Work out the finished part from the listing and answer in its coordinate system (mm). Coordinates: 2 decimals unless noted, no trailing zeros. Loops run counter-clockwise (first coordinate to the right, second up) from the corner with the lowest first, then second, coordinate; pieces in that order, holes last.
```python
from build123d import *

# Parameters (mm, degrees)
F1_DEPTH = 4.7625


with BuildPart() as f1:
    # F0 (on Front) → F1 (new body)
    with BuildSketch(Plane.XZ):
        with BuildLine():
            Line((-57.785, 0), (-2.54, 0))
            ThreePointArc((-2.54, 0), (-0.743949, 0.743949), (0, 2.54))
            Line((0, 2.54), (0, 35.56))
            ThreePointArc((0, 35.56), (-0.743949, 37.356051), (-2.54, 38.1))
            Line((-2.54, 38.1), (-10.16, 38.1))
            ThreePointArc((-10.16, 38.1), (-11.956051, 37.356051), (-12.7, 35.56))
            Line((-12.7, 35.56), (-12.7, 12.7))
            Line((-12.7, 12.7), (-17.4625, 12.7))
            Line((-17.4625, 12.7), (-17.4625, 35.56))
            ThreePointArc((-17.4625, 35.56), (-18.206449, 37.356051), (-20.0025, 38.1))
            Line((-20.0025, 38.1), (-40.3225, 38.1))
            ThreePointArc((-40.3225, 38.1), (-42.118551, 37.356051), (-42.8625, 35.56))
            Line((-42.8625, 35.56), (-42.8625, 12.7))
            Line((-42.8625, 12.7), (-47.625, 12.7))
            Line((-47.625, 12.7), (-47.625, 63.5))
            Line((-47.625, 63.5), (-47.625, 69.85))
            ThreePointArc((-47.625, 69.85), (-49.484872, 74.340128), (-53.975, 76.2))
            Line((-53.975, 76.2), (-78.359, 76.2))
            Line((-78.359, 76.2), (-84.709, 76.2))
            ThreePointArc((-84.709, 76.2), (-89.199128, 74.340128), (-91.059, 69.85))
            Line((-91.059, 69.85), (-91.059, 63.5))
            Line((-91.059, 63.5), (-91.059, 46.99))
            ThreePointArc((-91.059, 46.99), (-90.315051, 45.193949), (-88.519, 44.45))
            Line((-88.519, 44.45), (-80.899, 44.45))
            ThreePointArc((-80.899, 44.45), (-79.102949, 45.193949), (-78.359, 46.99))
            Line((-78.359, 46.99), (-78.359, 63.5))
            Line((-78.359, 63.5), (-60.325, 63.5))
            Line((-60.325, 63.5), (-60.325, 2.54))
            ThreePointArc((-60.325, 2.54), (-59.581051, 0.743949), (-57.785, 0))
        make_face()
    extrude(amount=F1_DEPTH)


solid = f1.part
```
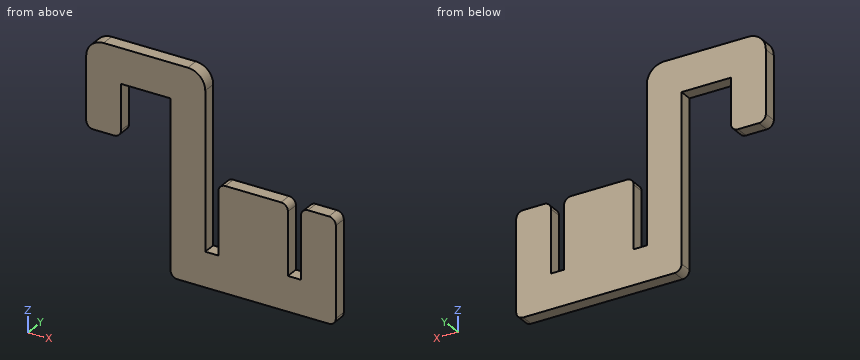
1. Each of these flat-tipped pins is pushed along its axis until it touches: P1, Ø2, axis at x = -58.5, z = 51, coming from the +Y side; P2, Ø2.5, axis at x = -68.5, y = -2, coming from the -Z side; P3, Ø1.5, axis at y = -1, z = 61.5, coming from the +X side (3 decimals); P4, Ø1.4, axis at x = -33.5, y = -1.5, coming from the +Z side. Where does it stop, or does it pass through?
2. A cutting plane is placed at D-D, the plane x = -16. Give the vertices of the cut face in (y, z), then the cut area to 3 significant figures.
3. A cutting plane is placed at B-B, the plane z = 27. Give the vertices of the cut face in (x, y) (1 decimal).
4. A cutting plane is placed at A-A, the plane z = 52. Give the vertices of the cut face in (x, y) (1 decimal).
5. Straight lines are drawn through the part: probe 1 along X at (y, z) = (-3.4, 34.5) (1 decimal); probe 2 along X at (y, z) = (-0.9, 50.5) (3 decimals); probe 3 along Z at (x, y) = (-64, -3.95). For each, find the intervals that lie inside material, in ascending order.
Answers below:
1. P1: stops at y = 0
1. P2: stops at z = 63.5
1. P3: stops at x = -47.625
1. P4: stops at z = 38.1
2. outline: (-4.76, 0) - (0, 0) - (0, 12.7) - (-4.76, 12.7) - close
2. area: 60.5 mm2
3. outline: (-60.3, -4.8) - (-47.6, -4.8) - (-47.6, 0) - (-60.3, 0) - close; (-42.9, -4.8) - (-17.5, -4.8) - (-17.5, 0) - (-42.9, 0) - close; (-12.7, -4.8) - (0, -4.8) - (0, 0) - (-12.7, 0) - close
4. outline: (-91.1, -4.8) - (-78.4, -4.8) - (-78.4, 0) - (-91.1, 0) - close; (-60.3, -4.8) - (-47.6, -4.8) - (-47.6, 0) - (-60.3, 0) - close
5. probe 1: x = -60.3 to -47.6, -42.9 to -17.5, -12.7 to 0
5. probe 2: x = -91.059 to -78.359, -60.325 to -47.625
5. probe 3: z = 63.5 to 76.2
